The model under review builds one solid part; all positions refer to its coordinate system, in mm. Face numbers are marked on the shaded views. A direction names the side the tool comes from. Round coordinates to 2 decimals unless told otherwise and drop trailing zeros. Write each loop counter-clockwise with the first axis right and the second up, starting at its lowest first coordinate (ties: lowest second). Pieces come first, ordered by that corner, then holes. Notation, with made-up numbers: (-14, 84.5) - (-9, 84.5) arc R35 cw to (-9, 119.5) - close; hole circle Ø3 at (19, -29). An arc over 180 degrees is marked (long way). One line per question, with ' | ' between items. Start each with the question number.
```python
from build123d import *

# Parameters (mm, degrees)
BOSS_EXTRUDE1_DEPTH      = 9.525
SKETCH2_W                = 254
SKETCH2_H                = 9.525
BOSS_EXTRUDE2_DEPTH      = 67.056
SKETCH3_W                = 254
SKETCH3_H                = 9.525
BOSS_EXTRUDE3_DEPTH      = 177.8
CONVERT_SOLID1_START     = -127
CONVERT_SOLID1_DEPTH     = 254
CONVERT_SOLID1_2_DEPTH   = 254
FILLET3_R                = 6.35
F_5_16_CLEARANCE_HOLE1_D = 8.4328
F_1_4_CLEARANCE_HOLE2_D  = 6.7564


# Read off the part's stored shape, not the designer's step: Convert-Solid1
with BuildPart() as part:
    # Sketch1 → Boss-Extrude1 (new body)
    with BuildSketch(Plane(origin=(0, 0, 0), x_dir=(1, 0, 0), z_dir=(0, 1, 0))):
        with BuildLine():
            Line((-127, 76.2), (127, 76.2))
            Line((127, 76.2), (127, -89.969927212))
            Line((127, -89.969927212), (8.874905057, -58.318403417))
            ThreePointArc((8.874905057, -58.318403417), (0, -57.15), (-8.874905057, -58.318403417))
            Line((-8.874905057, -58.318403417), (-127, -89.969927212))
            Line((-127, -89.969927212), (-127, 76.2))
        make_face()
    extrude(amount=BOSS_EXTRUDE1_DEPTH)

    # Sketch2 → Boss-Extrude2 (add)
    with BuildSketch(Plane(origin=(0, 9.525, 0), x_dir=(1, 0, 0), z_dir=(0, 1, 0))):
        with Locations((0, 71.4375)):
            Rectangle(SKETCH2_W, SKETCH2_H)
    extrude(amount=BOSS_EXTRUDE2_DEPTH)

    # Sketch3 → Boss-Extrude3 (add)
    with BuildSketch(Plane.XY.offset(-66.675)):
        with Locations((0, 81.3435)):
            Rectangle(SKETCH3_W, SKETCH3_H)
    extrude(amount=-BOSS_EXTRUDE3_DEPTH)

    # Convert-Solid1 outline → Convert-Solid1 (cut)
    with BuildSketch(Plane.YZ.offset(CONVERT_SOLID1_START)):
        with BuildLine():
            ThreePointArc((70.231, -66.675), (81.456320151, -71.324679849), (86.106, -82.55))
            Line((86.106, -82.55), (86.106, -66.675))
            Line((86.106, -66.675), (70.231, -66.675))
        make_face()
        with BuildLine():
            Line((0, -76.2), (15.875, -76.2))
            ThreePointArc((15.875, -76.2), (4.649679849, -71.550320151), (0, -60.325))
            Line((0, -60.325), (0, -76.2))
        make_face()
    extrude(amount=CONVERT_SOLID1_DEPTH, mode=Mode.SUBTRACT)

    # Convert-Solid1 2 outline → Convert-Solid1 2 (add)
    with BuildSketch(Plane.YZ.offset(CONVERT_SOLID1_START)):
        with BuildLine():
            Line((9.525, -66.675), (15.875, -66.675))
            ThreePointArc((15.875, -66.675), (11.384871939, -64.815128061), (9.525, -60.325))
            Line((9.525, -60.325), (9.525, -66.675))
        make_face()
        with BuildLine():
            ThreePointArc((70.231, -76.2), (74.721128061, -78.059871939), (76.581, -82.55))
            Line((76.581, -82.55), (76.581, -76.2))
            Line((76.581, -76.2), (70.231, -76.2))
        make_face()
    extrude(amount=CONVERT_SOLID1_2_DEPTH)

    # Fillet3
    fillet3_edges = [part.edges().sort_by_distance(p)[0] for p in [
        (127, 4.7625, 89.969927212),
        (-127, 4.7625, 89.969927212),
        (-127, 81.3435, -244.475),
        (127, 81.3435, -244.475),
    ]]
    fillet(fillet3_edges, radius=FILLET3_R)

    # 5/16 Clearance Hole1 (through all)
    with Locations(Plane(origin=(0, 86.106, 0), x_dir=(1, 0, 0), z_dir=(0, 1, 0))):
        with Locations((-113.109375, 233.3625), (-55.165625, 233.3625), (-55.165625, 155.575), (-113.109375, 155.575), (113.109375, 155.575), (55.165625, 155.575), (55.165625, 233.3625), (113.109375, 233.3625)):
            Hole(F_5_16_CLEARANCE_HOLE1_D / 2)

    # 1/4 Clearance Hole2 (through all)
    with Locations(Plane(origin=(0, 9.525, 0), x_dir=(1, 0, 0), z_dir=(0, 1, 0))):
        with Locations((0, 0), (0, 44.45), (30.795863359, 17.78), (38.494829198, -22.225), (0, -44.45), (-38.494829198, -22.225), (-38.494829198, 22.225)):
            Hole(F_1_4_CLEARANCE_HOLE2_D / 2)


solid = part.part
```
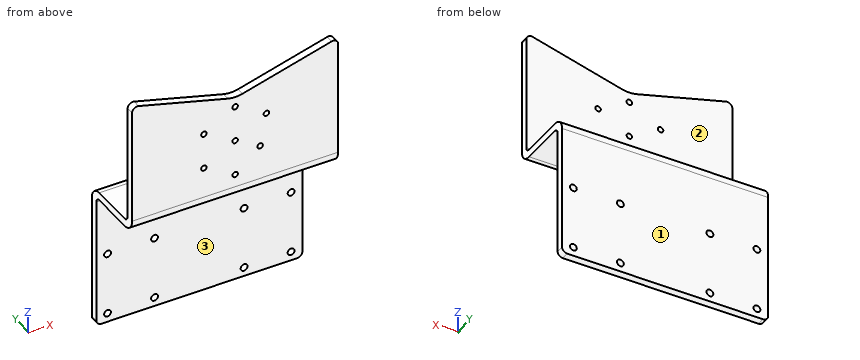
1. Machinability: for the marked faces 1, 2 and 3, which of the approach directions +Z, -Z, +X, -X, +Y, -Y give a long, thin tool a straight path to every point of the face, cutting with its end or side? Answer none if there is none.
2. Add section C-C, the plane x = -14. Write out the cut boundary in (y, z) (3 decimals).
3. Add section B-B, the plane z = -54.5. Write out the cut boundary in (x, y) (3 decimals).
4. Add section A-A, the plane y = 55. Write out the cut boundary in (x, z) (3 decimals).
5. Wall thickness on line 1 along Z through (x, y) = (0, 3); line 2 along X through (y, z) = (7, 44); line 3 along Y through (x, z) = (-91, 37) (3 decimals): over which ranges is each line inside the solid? List them lowest first. Write a range as [from, to].
6. Clearance check with flat-ended pins moving along their axes: P1, Ø9.5, axis at x = -113.11, z = -233.36, coming from the +Y side; P2, Ø16.5, axis at x = -33, y = 45, coming from the -Z side; P3, Ø11, axis at x = 113.11, z = -155.57, coming from the -Y side; P4, Ø1.5, axis at x = 46.5, z = 1, coming from the +Y side (3 decimals). State where each tip first meets the part, or that it passes through.
7. Add section D-D, the plane x = -69.5. Write out the cut boundary in (y, z) (3 decimals), then the cut area to 3 significant figures.
Geometry check:
1) face 1: +Z, -Z, +X, -X, +Y | face 2: +Z, +X, -X, +Y | face 3: -Z, +X, -X, -Y
2) outline: (0, -60.325) arc R15.875 ccw to (15.875, -76.2) - (70.231, -76.2) arc R6.35 cw to (76.581, -82.55) - (76.581, -244.475) - (86.106, -244.475) - (86.106, -82.55) arc R15.875 ccw to (70.231, -66.675) - (15.875, -66.675) arc R6.35 cw to (9.525, -60.325) - (9.525, 59.692) - (0, 59.692) - close
3) outline: (-127, 0) - (127, 0) - (127, 9.525) - (-127, 9.525) - close
4) outline: (-127, -76.2) - (127, -76.2) - (127, -66.675) - (-127, -66.675) - close
5) line 1: z = [-69.61, -47.83], [-41.07, -3.38], [3.38, 41.07], [47.83, 57.15] | line 2: x = [-127, -3.35], [3.35, 127] | line 3: y = [0, 9.525]
6) P1: stops at y = 86.11 | P2: stops at z = -76.2 | P3: stops at y = 76.58 | P4: stops at y = 9.525
7) outline: (0, -60.325) arc R15.875 ccw to (15.875, -76.2) - (70.231, -76.2) arc R6.35 cw to (76.581, -82.55) - (76.581, -244.475) - (86.106, -244.475) - (86.106, -82.55) arc R15.875 ccw to (70.231, -66.675) - (15.875, -66.675) arc R6.35 cw to (9.525, -60.325) - (9.525, 74.563) - (0, 74.563) - close | area: 3,680 mm2
